from build123d import *

# Parameters (mm, degrees)
SKETCH1_R                = 1.75
BOSS_EXTRUDE1_DEPTH      = 3.2
BOSS_EXTRUDE2_DEPTH      = 18
BOSS_EXTRUDE2_DEPTH_BACK = 6.4
CUT_EXTRUDE1_DEPTH       = 119.718371128
CUT_EXTRUDE1_DEPTH_BACK  = 3
SKETCH4_R                = 1.75
CHAMFER1_SIZE            = 2


with BuildPart() as part:
    # Sketch1 → Boss-Extrude1 (new, symmetric)
    with BuildSketch(Plane(origin=(0, 0, 0), x_dir=(1, 0, 0), z_dir=(0, 1, 0))):
        with BuildLine():
            Line((-14.064197212, 106.828183813), (-12.138935876, 92.204372108))
            ThreePointArc((-12.138935876, 92.204372108), (-8.327034738, 92.640714043), (-4.5, 92.914191088))
            Line((-4.5, 92.914191088), (-4.5, 90.60548378))
            Line((-4.5, 90.60548378), (-4.5, 89.092083998))
            Line((-4.5, 89.092083998), (-4.5, 87))
            ThreePointArc((-4.5, 87), (0, 82.5), (4.5, 87))
            Line((4.5, 87), (4.5, 89.092083998))
            Line((4.5, 89.092083998), (4.5, 90.60548378))
            Line((4.5, 90.60548378), (4.5, 92.914191088))
            ThreePointArc((4.5, 92.914191088), (8.327034738, 92.640714043), (12.138935876, 92.204372108))
            Line((12.138935876, 92.204372108), (14.064197212, 106.828183813))
            ThreePointArc((14.064197212, 106.828183813), (9.290945642, 107.337913445), (4.5, 107.638902983))
            Line((4.5, 107.638902983), (4.5, 109.907916002))
            Line((4.5, 109.907916002), (4.5, 112))
            ThreePointArc((4.5, 112), (0, 116.5), (-4.5, 112))
            Line((-4.5, 112), (-4.5, 109.907916002))
            Line((-4.5, 109.907916002), (-4.5, 107.638902983))
            ThreePointArc((-4.5, 107.638902983), (-9.290945642, 107.337913445), (-14.064197212, 106.828183813))
        make_face()
        with Locations(Location((0, 112, 0), (0, 0, 270))):
            Circle(SKETCH1_R, mode=Mode.SUBTRACT)
        with Locations(Location((0, 87, 0), (0, 0, 90))):
            Circle(SKETCH1_R, mode=Mode.SUBTRACT)
    extrude(amount=BOSS_EXTRUDE1_DEPTH, both=True)

    # Sketch3 → Boss-Extrude2 (add, two sides: drawn at the far end of the back side and taken through both)
    with BuildSketch(Plane(origin=(0, 3.2, 0), x_dir=(1, 0, 0), z_dir=(0, 1, 0)).offset(-BOSS_EXTRUDE2_DEPTH_BACK)):
        with BuildLine():
            Line((1.966607271, 94.760679154), (3.370522681, 105.424475409))
            ThreePointArc((3.370522681, 105.424475409), (2.956747146, 106.842837192), (1.636401853, 107.505897258))
            ThreePointArc((1.636401853, 107.505897258), (0, 107.524356631), (-1.636401853, 107.505897258))
            ThreePointArc((-1.636401853, 107.505897258), (-2.964387866, 106.850395337), (-3.385996272, 105.430720736))
            Line((-3.385996272, 105.430720736), (-1.982080861, 94.766924481))
            ThreePointArc((-1.982080861, 94.766924481), (-1.356871712, 93.547573592), (-0.06849064, 93.080907451))
            ThreePointArc((-0.06849064, 93.080907451), (0, 93.080930849), (0.06849064, 93.080907451))
            ThreePointArc((0.06849064, 93.080907451), (1.350413288, 93.544661639), (1.966607271, 94.760679154))
        make_face()
    extrude(amount=BOSS_EXTRUDE2_DEPTH + BOSS_EXTRUDE2_DEPTH_BACK)

    # Sketch4 → Cut-Extrude1 (cut, two sides: drawn at the far end of the back side and taken through both)
    # profile 1 of 2: a face of its own
    with BuildSketch(Plane(origin=(0, 3.2, 0), x_dir=(1, 0, 0), z_dir=(0, 1, 0)).offset(-CUT_EXTRUDE1_DEPTH_BACK)):
        with BuildLine():
            Line((-4.5, 91.393652938), (-4.5, 87.032555921))
            ThreePointArc((-4.5, 87.032555921), (0, 82.41632562), (4.5, 87.032555921))
            Line((4.5, 87.032555921), (4.5, 91.393652938))
            Line((4.5, 91.393652938), (4.5, 92.914191088))
            Line((4.5, 92.914191088), (-4.5, 92.914191088))
            Line((-4.5, 92.914191088), (-4.5, 91.393652938))
        make_face()
        with Locations(Location((0, 87, 0), (0, 0, 90))):
            Circle(SKETCH4_R, mode=Mode.SUBTRACT)
    # profile 2 of 2: a face of its own
    with BuildSketch(Plane(origin=(0, 3.2, 0), x_dir=(1, 0, 0), z_dir=(0, 1, 0)).offset(-CUT_EXTRUDE1_DEPTH_BACK)):
        with BuildLine():
            Line((4.5, 107.638902983), (-4.5, 107.638902983))
            Line((-4.5, 107.638902983), (-4.5, 112))
            ThreePointArc((-4.5, 112), (0, 116.5), (4.5, 112))
            Line((4.5, 112), (4.5, 107.638902983))
        make_face()
        with Locations(Location((0, 112, 0), (0, 0, 270))):
            Circle(SKETCH4_R, mode=Mode.SUBTRACT)
    extrude(amount=CUT_EXTRUDE1_DEPTH + CUT_EXTRUDE1_DEPTH_BACK, mode=Mode.SUBTRACT)

    # Chamfer1
    chamfer1_edges = [part.edges().sort_by_distance(p)[0] for p in [
        (0, 0.2, -85.25),
        (0, 0.2, -113.75),
    ]]
    chamfer(chamfer1_edges, length=CHAMFER1_SIZE)


solid = part.part
Read the model definition and answer for the solid it produces. Units are mm, in the model's axes. A direction names the side the tool comes from. Round coordinates to 2 decimals unless told otherwise and drop trailing zeros. Order: outer loops, then holes, each group sorted by start corner. A loop starts at its lowest first (then second) coordinate and runs counter-clockwise, first axis right, second up. Notation, with made-up numbers: (16, 52) - (23, 52) arc R14 ccw to (23, 71) - close; hole circle Ø11 at (0.25, 60). An arc over 180 degrees is marked (long way). Use one line per item in the form item = value. Start each with the question number.
(1) The part is cut by section C-C (z = -103). Give the vertices of the cut face in (x, y), then the cut area to 3 significant figures.
(2) The part is cut by section A-A (y = 11.5). Give the vertices of the cut face in (x, z), then the cut area to 4 significant figures.
(3) The part is cut by section B-B (x = -0.75). Count the separate pieces of the cut face and the enclosed holes in it, then the cut area to 3 significant figures.
(4) Flat-ended cylindrical pins translate along their axes: pin 1 Ø3.5 at (x, y) = (-1, 1.5) entering from +Z; pin 2 Ø4 at (x, y) = (4, 3) entering from +Z; pin 3 Ø4 at (y, z) = (1.5, -110.5) entering from -X; pin 4 Ø4 at (x, z) = (0, -112) entering from +Y. Find the tip coordinate at first contact, or state that the pin passes through.
(5) For faces 5 (the face through (0, 2, -107.639)), 6 (the face through (0, 0.2, -91)), 7 (the face through (2.66, 12.07, -100.02)), determine the directions among +Z, -Z, +X, -X, +Y, -Y from which every point of the face is accessible in a straight line to the end or side of a thin tool.
(6) Determine the mould class of faces 1 (the face through (3, 3.2, -100)), 2 (the face through (-4.5, -1, -110)), 3 (the face through (9.358, 0.045, -107.332)), 4 (the face through (0.526, -2.51, -110.331)) for opening direction X: +X half, -X half, draft (parallel to the pull), parting line (faces both ways), or undercut.
(7) Find the intervals of material crossed by line 1 along X through (y, z) = (-2.65, -87); line 2 along Y through (x, z) = (-6.5, -103); line 3 along Z through (x, y) = (2, 2.5), in increasing order. Write a range as from..to.
Checked values:
q1.outline = (-13.56, -3.2) - (13.56, -3.2) - (13.56, 3.2) - (3.05, 3.2) - (3.05, 21.2) - (-3.07, 21.2) - (-3.07, 3.2) - (-13.56, 3.2) - close
q1.area = 284 mm^2
q2.outline = (-3.39, -105.43) arc R1.85 ccw to (-1.64, -107.51) arc R72.54 ccw to (1.64, -107.51) arc R1.85 ccw to (3.37, -105.42) - (1.97, -94.76) arc R1.85 ccw to (0.07, -93.08) arc R100.24 cw to (-0.07, -93.08) arc R1.87 ccw to (-1.98, -94.77) - close
q2.area = 74.95 mm^2
q3.separate_pieces = 3
q3.enclosed_holes = 0
q3.area = 387 mm^2
q4.pin_1 = -82.5
q4.pin_2 = -92.83
q4.pin_3 = -4.5
q4.pin_4 = -1.55
q5.face_5 = -Z, +X, -X, +Y
q5.face_6 = +Z, +Y
q5.face_7 = +Z, +X, +Y
q6.face_1 = draft
q6.face_2 = -X half
q6.face_3 = +X half
q6.face_4 = undercut
q7.line_1 = -4.5..-1.75, 1.75..4.5
q7.line_2 = -3.2..3.2
q7.line_3 = -107.64..-92.91
